Check sheet for the drawn part. Datum: minimum x, y, z corner. Units: mm. A direction names the side the tool comes from. Coordinates: 2 decimals unless noted, no trailing zeros. Write each loop counter-clockwise with the first axis right and the second up, starting at its lowest first coordinate (ties: lowest second). Pieces come first, ordered by that corner, then holes. Notation, with made-up numbers: (27, 34.25) -> (79, 34.25) arc R29 ccw to (79, 57.25) -> close; hole circle Ø1 at (42, 79.5). An arc over 180 degrees is marked (long way). Answer in a Markdown table with one row per item. Add a question column.
Q1. Release check for a two-part mould opening along X. For the marked faces 4, 5 and 6 record: pulls with the +X half, pulls with the -X half, needs draft (parallel to the pull), parting line crosses it, or undercut.
Q2. Section check B-B, the plane x = 5.5. Record the boundary of the cut face in (y, z) (1 decimal).
Q3. Tool access check on the marked faces 1, 2 and 3. Record the directions out of +Z, -Z, +X, -X, +Y, -Y that give a thin tool (end or side, any length) a straight path to the whole face; none if there is none.
Q4. Section check A-A, the plane z = 2.25. Record the boundary of the cut face in (x, y) (1 decimal).
Q5. Section check D-D, the plane z = 13.75. Record the boundary of the cut face in (x, y).
Q6. Gauge pin test, flat ends, axial feed: P1, Ø2, axis at x = 2, z = 2, coming from the -Y side; P2, Ø0.9, axis at y = 3, z = 1.5, coming from the -X side. Record the tip position at first contact, or that the pin passes through.
Q7. Thickness scan on line 1 (Z direction, x = 4.5, y = 2.5) (1 decimal); line 2 (Z direction, x = 2, y = 2); line 3 (X direction, y = 3.5, z = 2) (1 decimal). Record the ranges inside material, lowest first.
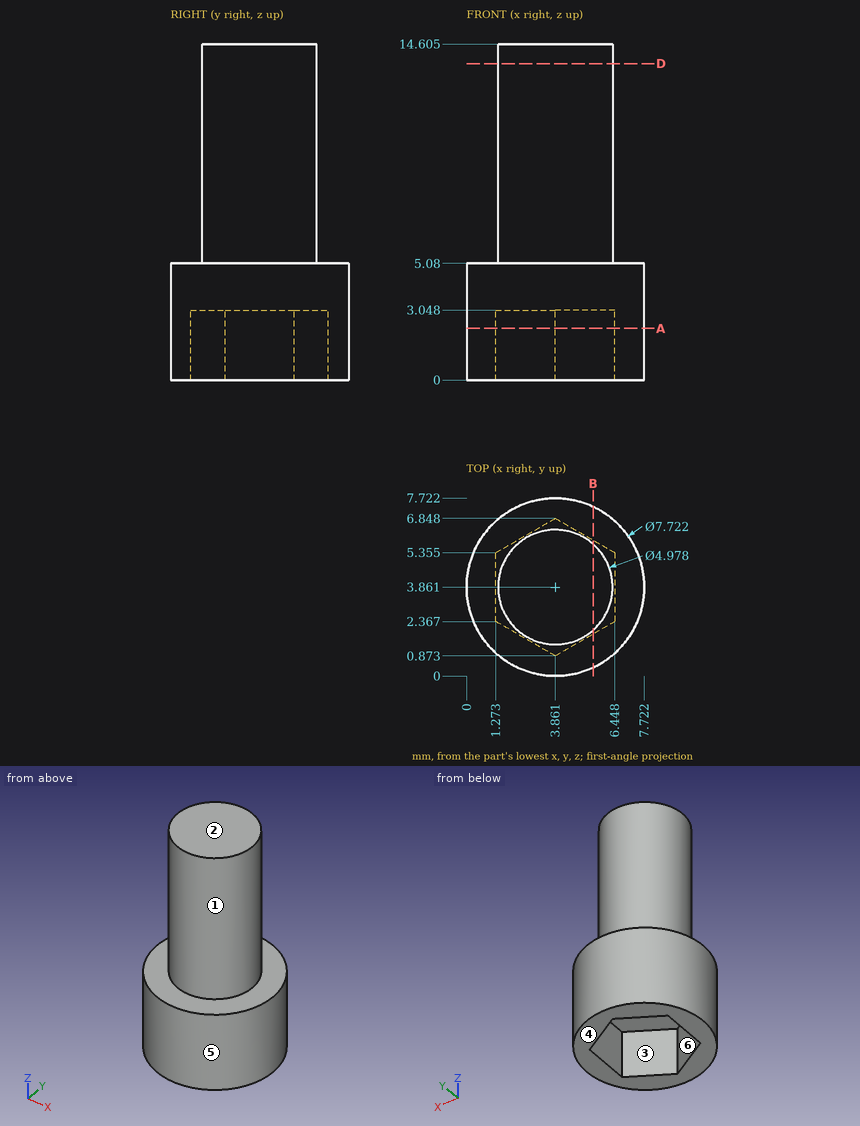
Calculated:
| question | item | result |
|---|---|---|
| 1 | face 4 | needs draft |
| 1 | face 5 | parting line crosses it |
| 1 | face 6 | undercut |
| 2 | outline | (0.4, 0) -> (1.8, 0) -> (1.8, 3) -> (5.9, 3) -> (5.9, 0) -> (7.4, 0) -> (7.4, 5.1) -> (5.7, 5.1) -> (5.7, 14.6) -> (2, 14.6) -> (2, 5.1) -> (0.4, 5.1) -> close |
| 3 | face 1 | +Z |
| 3 | face 2 | +Z, +X, -X, +Y, -Y |
| 3 | face 3 | -Z |
| 4 | outline | circle Ø7.7 at (3.9, 3.9); hole (1.3, 2.4) -> (3.9, 0.9) -> (6.4, 2.4) -> (6.4, 5.4) -> (3.9, 6.8) -> (1.3, 5.4) -> close |
| 5 | outline | circle Ø4.98 at (3.86, 3.86) |
| 6 | P1 | stops at y = 0.1 |
| 6 | P2 | stops at x = 0.02 |
| 7 | line 1 | z = 3 to 14.6 |
| 7 | line 2 | z = 3.05 to 5.08 |
| 7 | line 3 | x = 0 to 1.3, 6.4 to 7.7 |
